Can you work these out from the model? Positions are in its coordinate system, mm. A direction names the side the tool comes from. Coordinates: 2 decimals unless noted, no trailing zeros. Order: outer loops, then holes, each group sorted by start corner. A loop starts at its lowest first (then second) coordinate and runs counter-clockwise, first axis right, second up. Notation, with made-up numbers: (-24, -35.5) -> (-5, -35.5) arc R36 ccw to (-5, -0.5) -> close; hole circle Ø3 at (70, 4.25). An arc over 180 degrees is marked (long way). Answer as a JSON object with one key per item and string values. Group by question number.
(1) For pin 1 (3 mm diameter, centred on x = -2.5, z = 8, fed in from -Y); pin 2 (11 mm diameter, centred on x = 0, y = 0, fed in from -Z), each with a flat end and sliding along its axis, tell me the tip position at first contact or that it passes through.
(2) I want a section at A-A, the plane x = 0. List the corners of the cut face in (y, z) for me, plus the area to 3 significant figures.
(3) If we mould it in two halves opening along Y, with no side actions, what happens to faces 1 (the cylindrical face through (10.07, 62.5, 11.63)), 2 (the flat face through (-5.2, 49, 13)), 3 (the cylindrical face through (10.9, 29.91, 0.57)), 4 (the flat face through (-0.087, 56.893, 1.393))? For each: pulls with the +Y half, pulls with the -Y half, needs draft (parallel to the pull), parting line crosses it, or undercut.
(4) I want a section at C-C, the plane z = 12. List the corners of the cut face in (x, y) for me, plus the area to 3 significant figures.
(5) I want a section at B-B, the plane y = 52. List the corners of the cut face in (x, z) for me, plus the area to 3 significant figures.
(6) Which directions (+Z, -Z, +X, -X, +Y, -Y) give clear straight access to the entire face, cutting with the end or side of a thin tool? Please do faces 5 (the flat face through (0, 56.4, 13)), 6 (the flat face through (11.5, 29, 11)), 7 (the flat face through (-0.087, 40.507, 1.393)).
(7) I need wall thicknesses on line 1 (Y direction, x = 0, z = 7.5); line 2 (Y direction, x = -2.5, z = 13.25); line 3 (Z direction, x = 9.75, y = 30). Which ranges of each line are inside material? Lowest first, please.
(8) I want a section at D-D, the plane y = 2.5. List the corners of the cut face in (x, z) for me.
from build123d import *

# Parameters (mm, degrees)
SKETCH1_W           = 10.4
SKETCH1_H           = 15.4
SKETCH1_R           = 11.5
SKETCH1_R_2         = 6.25
BOSS_EXTRUDE1_DEPTH = 23
CHAMFER2_SIZE       = 1
CHAMFER2_SIZE2      = 2.747477419
FILLET2_R           = 5
FILLET3_R           = 2


with BuildPart() as part:
    # Sketch1 → Boss-Extrude1 (new body)
    # profile 1 of 2: a face of its own
    with BuildSketch(Plane.XY):
        with BuildLine():
            Line((-11.5, 64), (-11.5, 4e-09))
            ThreePointArc((-11.5, 4e-09), (2e-09, 11.5), (11.5, 0))
            Line((11.5, 0), (11.5, 64))
            Line((11.5, 64), (-11.5, 64))
        make_face()
        with Locations((0, 48.7)):
            Rectangle(SKETCH1_W, SKETCH1_H, mode=Mode.SUBTRACT)
    # profile 2 of 2: a face of its own
    with BuildSketch(Plane.XY):
        Circle(SKETCH1_R)
        Circle(SKETCH1_R_2, mode=Mode.SUBTRACT)
    extrude(amount=BOSS_EXTRUDE1_DEPTH)

    # Chamfer2
    chamfer2_edges = [part.edges().sort_by_distance(p)[0] for p in [
        (0, 56.4, 0),
        (-5.2, 48.7, 0),
        (0, 41, 0),
        (5.2, 48.7, 0),
    ]]
    chamfer2_side = [part.faces().sort_by_distance(p)[0] for p in [
        (0, 27.411701329, 0),
    ]]
    chamfer(chamfer2_edges, length=CHAMFER2_SIZE, length2=CHAMFER2_SIZE2, reference=chamfer2_side[0])

    # Fillet2
    fillet2_edges = [part.edges().sort_by_distance(p)[0] for p in [
        (-11.5, 64, 11.5),
        (11.5, 64, 11.5),
    ]]
    fillet(fillet2_edges, radius=FILLET2_R)

    # Fillet3
    fillet3_edges = [part.edges().sort_by_distance(p)[0] for p in [
        (-2e-09, -11.5, 23),
        (11.5, 29.5, 0),
        (-2e-09, -11.5, 0),
        (-11.5, 29.500000002, 0),
        (11.5, 29.5, 23),
        (0, 64, 0),
        (10.035533906, 62.535533906, 0),
        (-10.035533906, 62.535533906, 0),
        (0, 64, 23),
        (10.035533906, 62.535533906, 23),
        (-10.035533906, 62.535533906, 23),
        (-11.5, 29.500000002, 23),
    ]]
    fillet(fillet3_edges, radius=FILLET3_R)


solid = part.part
Computed values:
{
 "1": {"pin 1": "stops at y = -11.46", "pin 2": "passes through"},
 "2": {"outline": "(-11.5, 2) arc R2 ccw to (-9.5, 0) -> (-6.25, 0) -> (-6.25, 23) -> (-9.5, 23) arc R2 ccw to (-11.5, 21) -> close; (6.25, 0) -> (40, 0) -> (41, 2.75) -> (41, 23) -> (6.25, 23) -> close; (56.4, 2.75) -> (57.4, 0) -> (62, 0) arc R2 ccw to (64, 2) -> (64, 21) arc R2 ccw to (62, 23) -> (56.4, 23) -> close", "area": "1,090 mm2"},
 "3": {"face 1": "pulls with the +Y half", "face 2": "undercut", "face 3": "needs draft", "face 4": "undercut"},
 "4": {"outline": "(-11.5, 0) arc R11.5 ccw to (11.5, 0) -> (11.5, 59) arc R5 ccw to (6.5, 64) -> (-6.5, 64) arc R5 ccw to (-11.5, 59) -> close; hole circle Ø12.5 at (0, 0); hole (-5.2, 41) -> (5.2, 41) -> (5.2, 56.4) -> (-5.2, 56.4) -> close", "area": "1,390 mm2"},
 "5": {"outline": "(-11.5, 2) arc R2 ccw to (-9.5, 0) -> (-6.2, 0) -> (-5.2, 2.75) -> (-5.2, 23) -> (-9.5, 23) arc R2 ccw to (-11.5, 21) -> close; (5.2, 2.75) -> (6.2, 0) -> (9.5, 0) arc R2 ccw to (11.5, 2) -> (11.5, 21) arc R2 ccw to (9.5, 23) -> (5.2, 23) -> close", "area": "284 mm2"},
 "6": {"face 5": "+Z, -Z", "face 6": "+Z, -Z, +X, +Y, -Y", "face 7": "-Z"},
 "7": {"line 1": "y = -11.5 to -6.25, 6.25 to 41, 56.4 to 64", "line 2": "y = -11.22 to -5.73, 5.73 to 41, 56.4 to 64", "line 3": "z = 0.02 to 22.98"},
 "8": {"outline": "(-11.5, 2) arc R2 ccw to (-9.5, 0) -> (-5.73, 0) -> (-5.73, 23) -> (-9.5, 23) arc R2 ccw to (-11.5, 21) -> close; (5.73, 0) -> (9.5, 0) arc R2 ccw to (11.5, 2) -> (11.5, 21) arc R2 ccw to (9.5, 23) -> (5.73, 23) -> close"}
}
